Could you check a few things on this model? Use its own coordinates, in mm. A direction names the side the tool comes from. Coordinates: 2 decimals unless noted, no trailing zeros. Write each loop counter-clockwise with the first axis right and the second up, starting at its lowest first coordinate (ties: lowest second). Pieces come first, ordered by that corner, then holes.
```python
from build123d import *

# Parameters (mm, degrees)
F1_DEPTH = 25
F2_R     = 1.5
F3_DEPTH = 36.001
F4_R     = 2.145417
F5_DEPTH = 50.001
F6_R     = 2.624868
F7_DEPTH = 36.001


with BuildPart() as f1:
    # F0 (on Front) → F1 (new body)
    with BuildSketch(Plane.XZ):
        Polygon((25, 18), (-25, 18), (-25, -18), (25, -18), (25, -14), (22.5, -14), (-22.5, -14), (-22.5, 14), (22.5, 14), (25, 14), align=None)
    extrude(amount=F1_DEPTH)

    # F2 (on face) → F3 (cut, through all)
    with BuildSketch(Plane.XY.offset(18)):
        with Locations((17.761598, -12.5)):
            Circle(F2_R)
    extrude(amount=-F3_DEPTH, mode=Mode.SUBTRACT)

    # F4 (on face) → F5 (cut, through all)
    with BuildSketch(Plane(origin=(-25, 0, 0), x_dir=(0, -1, 0), z_dir=(-1, 0, 0))):
        with Locations((12.5, 0)):
            Circle(F4_R)
    extrude(amount=-F5_DEPTH, mode=Mode.SUBTRACT)

    # F6 (on face) → F7 (cut, through all)
    with BuildSketch(Plane.XY.offset(18)):
        with Locations((-7.933488, -12.5)):
            Circle(F6_R)
    extrude(amount=-F7_DEPTH, mode=Mode.SUBTRACT)


solid = f1.part
```
Item 1: I want a section at B-B, the plane x = 6. List the corners of the cut face in (y, z) for me.
Item 2: If we mould it in two halves opening along X, with no side actions, what happens to faces 1 (the cylindrical face through (19.192, -12.049, 16.028)), 2 (the flat face through (25, -12, -16)), 3 (the flat face through (1, -12, 14))? For each: released by +X, released by -X, zero draft, split by the parting line, or undercut.
Item 3: I want a section at C-C, the plane y = -12.5. List the corners of the cut face in (x, z) for me.
Item 4: If I drill on line 1 along Z through (x, y) = (6.5, -18); line 2 along X through (y, z) = (-23, -2); line 3 along Z through (x, y) = (-23.9, -12.5), over which ranges is the centre line in solid material (lowest first)?
Item 5: I want a section at D-D, the plane y = -18.5. List the corners of the cut face in (x, z) for me.
Item 6: Will this pin go through, and if not, where does the flat tip stop? pin 1 Ø5.5 at (y, z) = (-12.5, 0) entering from +X.
Item 7: Which directions (+Z, -Z, +X, -X, +Y, -Y) give clear straight access to the entire face, cutting with the end or side of a thin tool? Please do faces 4 (the cylindrical face through (-23.768, -10.357, 0.094)), 5 (the flat face through (-22.5, -10, 0)).
Item 8: I want a section at A-A, the plane z = 0. List the corners of the cut face in (x, y) for me.
Taken from the geometry:
1. outline: (-25, -18) - (0, -18) - (0, -14) - (-25, -14) - close; (-25, 14) - (0, 14) - (0, 18) - (-25, 18) - close
2. face 1: undercut
2. face 2: released by +X
2. face 3: zero draft
3. outline: (-25, -18) - (-10.56, -18) - (-10.56, -14) - (-22.5, -14) - (-22.5, -2.15) - (-25, -2.15) - close; (-25, 2.15) - (-22.5, 2.15) - (-22.5, 14) - (-10.56, 14) - (-10.56, 18) - (-25, 18) - close; (-5.31, -18) - (16.26, -18) - (16.26, -14) - (-5.31, -14) - close; (-5.31, 14) - (16.26, 14) - (16.26, 18) - (-5.31, 18) - close; (19.26, -18) - (25, -18) - (25, -14) - (19.26, -14) - close; (19.26, 14) - (25, 14) - (25, 18) - (19.26, 18) - close
4. line 1: z = -18 to -14, 14 to 18
4. line 2: x = -25 to -22.5
4. line 3: z = -18 to -2.15, 2.15 to 18
5. outline: (-25, -18) - (25, -18) - (25, -14) - (-22.5, -14) - (-22.5, 14) - (25, 14) - (25, 18) - (-25, 18) - close
6. pin 1: stops at x = -22.5
7. face 4: +X, -X
7. face 5: +X, +Y, -Y
8. outline: (-25, -25) - (-22.5, -25) - (-22.5, -14.65) - (-25, -14.65) - close; (-25, -10.35) - (-22.5, -10.35) - (-22.5, 0) - (-25, 0) - close
